Could you check a few things on this drawing? It's one solid part, dimensions in mm from its lowest x, y, z. Round coordinates to 2 decimals unless told otherwise and drop trailing zeros. Loops run counter-clockwise (first coordinate to the right, second up) from the corner with the lowest first, then second, coordinate; pieces in that order, holes last. Notation, with made-up numbers: M 34,28 L 69,28 A30 ccw 69,57 Z; hole C 80,55 d3. An arc over 180 degrees is marked long. Write each question's results on one line, items separated by ' | '. Start each with the question number.
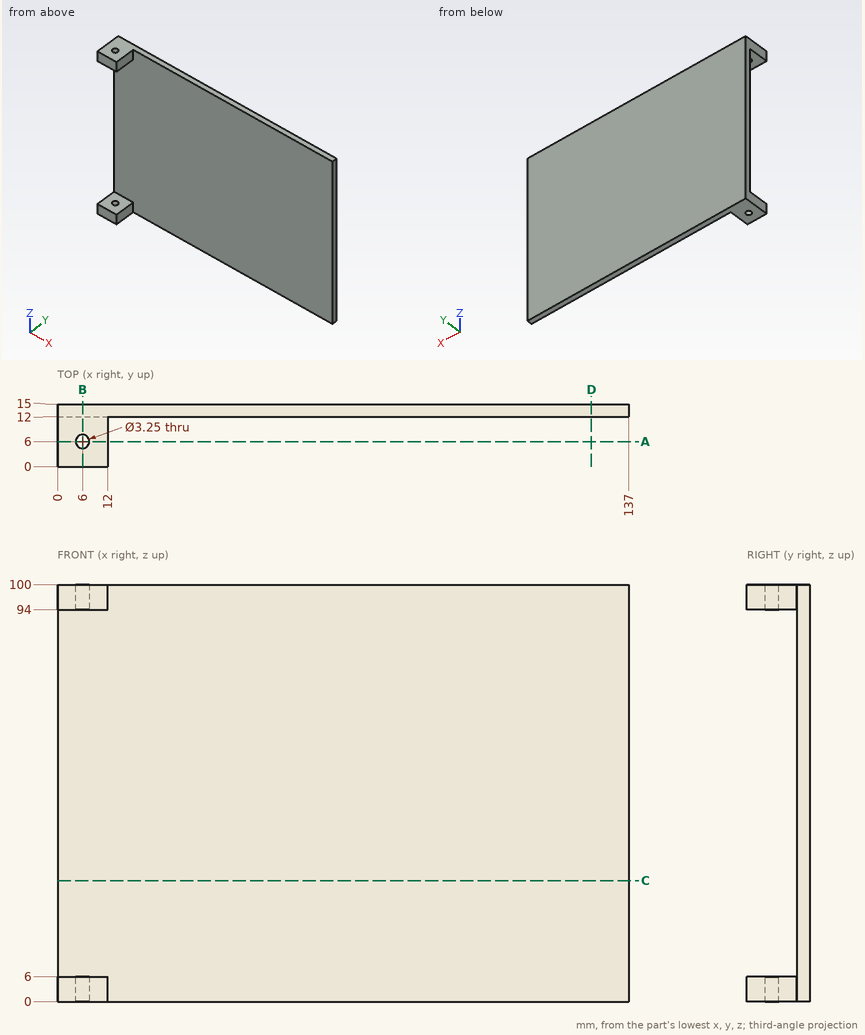
1. I want a section at D-D on x = 128. List the corners of the cut face in (y, z) for me, plus the area to 3 significant figures.
2. I want a section at B-B on x = 6. List the corners of the cut face in (y, z) for me (3 decimals), plus the area to 3 significant figures.
3. I want a section at A-A on y = 6. List the corners of the cut face in (x, z) for me (3 decimals).
4. I need wall thicknesses on line 1 along Y through (x, z) = (6, 95.35) (3 decimals); line 2 along Y through (x, z) = (91, 28); line 3 along X through (y, z) = (2.25, 4). Which ranges of each line are inside material? Lowest first, please.
5. For pin 1 (1.9 mm diameter, centred on x = 6, y = 6, fed in from +Z); pin 2 (1.8 mm diameter, centred on y = 5, z = 96.5, fed in from +X), each with a flat end and sliding along its axis, tell me the tip position at first contact or that it passes through.
6. I want a section at C-C on z = 29. List the corners of the cut face in (x, y) for me.
Outcome:
1) outline: M 12,0 L 15,0 L 15,100 L 12,100 Z | area: 300 mm2
2) outline: M 0,0 L 4.375,0 L 4.375,6 L 0,6 Z; M 0,94 L 4.375,94 L 4.375,100 L 0,100 Z; M 7.625,0 L 15,0 L 15,100 L 7.625,100 L 7.625,94 L 12,94 L 12,6 L 7.625,6 Z | area: 405 mm2
3) outline: M 0,0 L 4.375,0 L 4.375,6 L 0,6 Z; M 0,94 L 4.375,94 L 4.375,100 L 0,100 Z; M 7.625,0 L 12,0 L 12,6 L 7.625,6 Z; M 7.625,94 L 12,94 L 12,100 L 7.625,100 Z
4) line 1: 0 to 4.375, 7.625 to 15 | line 2: 12 to 15 | line 3: 0 to 12
5) pin 1: through | pin 2: x = 12
6) outline: M 0,12 L 137,12 L 137,15 L 0,15 Z
